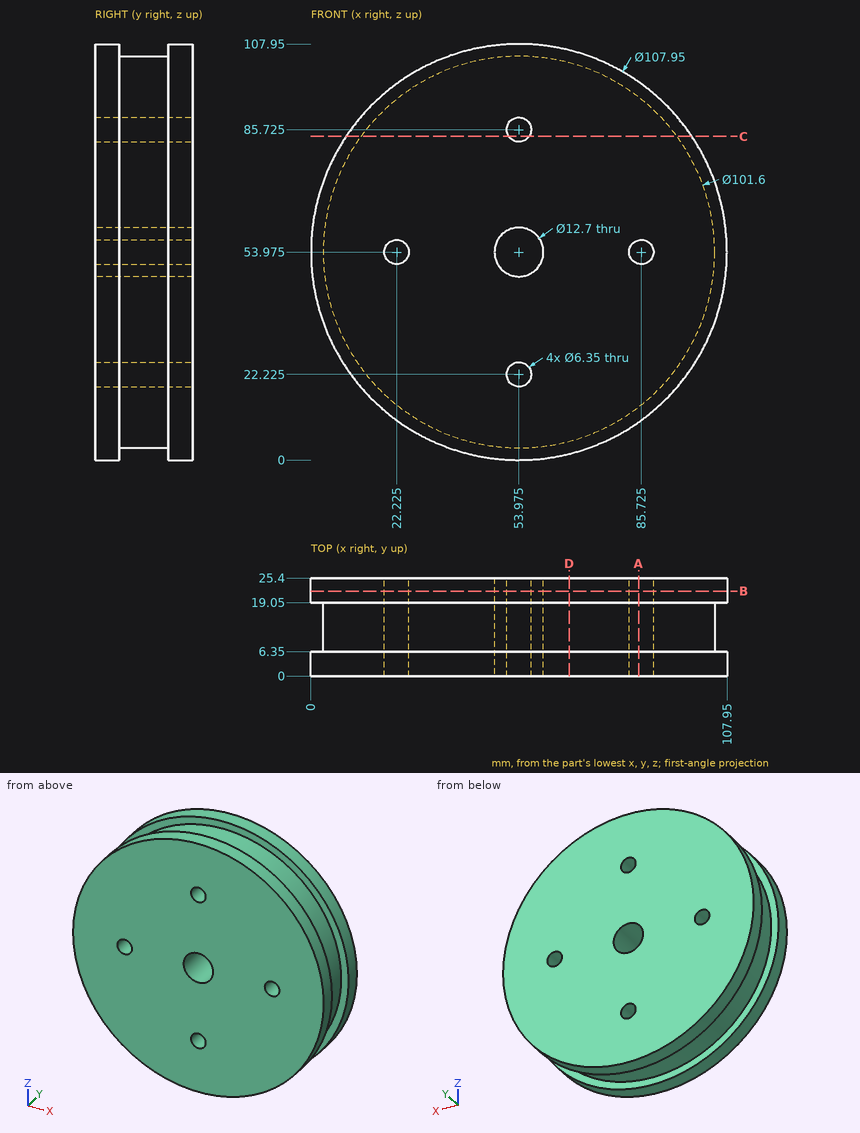
For this review, use the dimensioned drawing (mm, ordinates from the lowest corner) and the shaded views. Coordinates: 2 decimals unless noted, no trailing zeros. Order: outer loops, then holes, each group sorted by start corner. A loop starts at its lowest first (then second) coordinate and runs counter-clockwise, first axis right, second up. Notation, with made-up numbers: M 7.25,-35 L 52.25,-35 A22 ccw 52.25,2 Z; hole C 52,77 d3. An arc over 180 degrees is marked long. Answer as a JSON object with one key per item and string values. Group by question number.
1) Wall thickness on L1, parallel to Y at x = 88, z = 13.5; L2, parallel to Z at x = 49, y = 5.5; L3, parallel to X at y = 17.25, z = 86: over which ranges is each line inside the solid? List them lowest first.
2) For pin 1 (4 mm diameter, centred on y = 13.5, z = 63, fed in from -X); pin 2 (5 mm diameter, centred on x = 19, y = 11.5, fed in from +Z); pin 3 (6 mm diameter, centred on x = 37, y = 19, fed in from +Z), all flat-tipped, find the tip position at first contact; note any pin that passes through.
3) Add section D-D, the plane x = 67. Write out the cut boundary in (y, z), then the cut area to 3 significant figures.
4) Add section A-A, the plane x = 85. Write out the cut boundary in (y, z).
5) Add section C-C, the plane z = 84. Write out the cut boundary in (x, y).
6) Add section B-B, the plane y = 22. Write out the cut boundary in (x, z) (3 decimals).
Computed values:
{
 "1": {"L1": "y = 0 to 6.35, 19.05 to 25.4", "L2": "z = 0.23 to 50.03, 57.92 to 107.72", "L3": "x = 14.54 to 50.81, 57.14 to 93.41"},
 "2": {"pin 1": "stops at x = 3.66", "pin 2": "stops at z = 93.04", "pin 3": "stops at z = 106.11"},
 "3": {"outline": "M 0,1.6 L 6.35,1.6 L 6.35,4.87 L 19.05,4.87 L 19.05,1.6 L 25.4,1.6 L 25.4,106.35 L 19.05,106.35 L 19.05,103.08 L 6.35,103.08 L 6.35,106.35 L 0,106.35 Z", "area": "2,580 mm^2"},
 "4": {"outline": "M 0,9.81 L 6.35,9.81 L 6.35,13.75 L 19.05,13.75 L 19.05,9.81 L 25.4,9.81 L 25.4,50.88 L 0,50.88 Z; M 0,57.07 L 25.4,57.07 L 25.4,98.14 L 19.05,98.14 L 19.05,94.2 L 6.35,94.2 L 6.35,98.14 L 0,98.14 Z"},
 "5": {"outline": "M 9.12,0 L 51.31,0 L 51.31,25.4 L 9.12,25.4 L 9.12,19.05 L 13,19.05 L 13,6.35 L 9.12,6.35 Z; M 56.64,0 L 98.83,0 L 98.83,6.35 L 94.95,6.35 L 94.95,19.05 L 98.83,19.05 L 98.83,25.4 L 56.64,25.4 Z"},
 "6": {"outline": "C 53.975,53.975 d107.95; hole C 22.225,53.975 d6.35; hole C 53.975,53.975 d12.7; hole C 53.975,22.225 d6.35; hole C 53.975,85.725 d6.35; hole C 85.725,53.975 d6.35"}
}
